Autodesk Inventor part; units mm, degrees
ref_plane "YZ Plane" through (0, 0, 0) normal (1, 0, 0) x (0, 1, 0)
ref_plane "XZ Plane" through (0, 0, 0) normal (0, 1, 0) x (-1, 0, 0)
ref_plane "XY Plane" through (0, 0, 0) normal (0, 0, 1) x (1, 0, 0)
sketch "Sketch1" plane through (0, 0, 0) normal (0, 1, 0) x (-1, 0, 0)
  line L0 (15.3914, 31.136) -> (0.1514, 31.136)
  line L1 (0.1514, 31.136) -> (0.1514, 15.896)
  line L2 (0.1514, 15.896) -> (15.3914, 15.896)
  line L3 (15.3914, 15.896) -> (15.3914, 31.136)
  point P0 (0, 0)
  dimension "d0" = 15.24
  dimension "d1" = 15.24
extrude "Extrusion1" add sketch "Sketch1" along normal blind 7.62
sketch "Sketch2" plane through (0, 0, 0) normal (0, -1, 0) x (1, 0, 0)
  circle A0 centre (-7.8533, 23.6101) radius 3.7937
  point P0 (0, 0)
extrude "Extrusion2" add sketch "Sketch2" along normal blind 1.778
sketch "Sketch3" plane through (0, 0, 0) normal (0, -1, 0) x (1, 0, 0)
  circle A0 centre (-1.4346, 30.0524) radius 0.8632
  circle A1 centre (-1.4346, 16.9205) radius 0.8792
  circle A2 centre (-14.354, 30.0524) radius 0.8098
  circle A3 centre (-14.354, 16.9205) radius 0.7609
  point P0 (0, 0)
extrude "Extrusion3" add sketch "Sketch3" along normal blind 0.508
sketch "Sketch4" plane through (0, 7.62, 0) normal (0, 1, 0) x (1, 0, 0)
  line L0 (-15.3914, -15.896) -> (-15.3914, -31.136)
  line L1 (-15.3914, -31.136) -> (-14.9868, -31.136)
  line L2 (-14.9868, -31.136) -> (-14.9868, -30.723)
  line L3 (-14.9868, -30.723) -> (-15.3914, -30.723)
  line L4 (-15.3914, -30.723) -> (-15.3914, -31.136)
  line L5 (-0.1514, -15.896) -> (-15.3914, -15.896)
  line L6 (-15.3914, -15.896) -> (-14.9868, -15.896)
  line L7 (-14.9868, -15.896) -> (-14.9868, -16.2998)
  line L8 (-14.9868, -16.2998) -> (-15.3914, -16.2998)
  line L9 (-15.3914, -16.2998) -> (-15.3914, -15.896)
  line L10 (-0.1514, -15.896) -> (-0.5623, -15.896)
  line L11 (-0.5623, -15.896) -> (-0.5623, -16.3119)
  line L12 (-0.5623, -16.3119) -> (-0.1514, -16.3119)
  line L13 (-0.1514, -16.3119) -> (-0.1514, -15.896)
  line L14 (-15.3914, -31.136) -> (-0.1514, -31.136)
  line L15 (-0.1514, -31.136) -> (-0.5623, -31.136)
  line L16 (-0.5623, -31.136) -> (-0.5623, -30.723)
  line L17 (-0.5623, -30.723) -> (-0.1514, -30.723)
  line L18 (-0.1514, -30.723) -> (-0.1514, -31.136)
  point P0 (0, 0)
extrude "Extrusion4" add sketch "Sketch4" along normal blind 6.35
properties part number "switch"
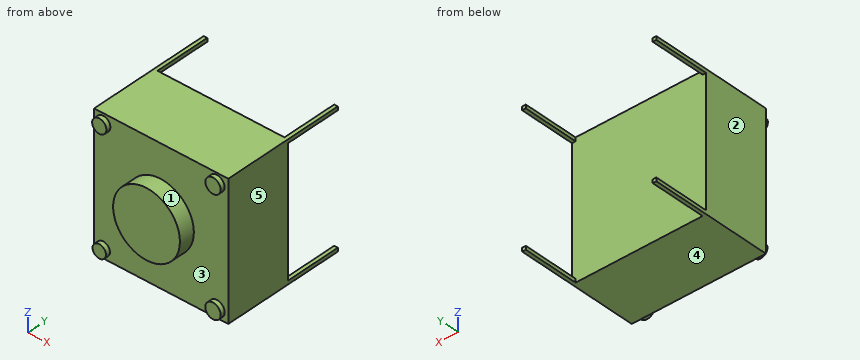
Work out the finished part from the listing and answer in its coordinate system (mm). Face numbers are marked on the shaded views. A direction names the side the tool comes from. Round coordinates to 2 decimals unless told otherwise and drop trailing zeros. Write each loop counter-clockwise with the first axis right and the second up, starting at its lowest first coordinate (ties: lowest second). Pieces come first, ordered by that corner, then holes. Notation, with made-up numbers: (87, 6.25) -> (112, 6.25) arc R29 ccw to (112, 38.25) -> close; hole circle Ø4 at (-25.5, 85.25). An arc over 180 degrees is marked (long way). Write each question's results on one line, items separated by ' | '.
Item 1: Which of the six approach directions +Z, -Z, +X, -X, +Y, -Y give full straight-line access (tool end or side, diameter ignored) to the marked faces 1 and 2?
Result set:
face 1: -Y | face 2: +Z, -Z, -X, +Y, -Y
Item 2: A cutting plane is placed at B-B, the plane x = -7.5. Determine the outline of the cut face in (y, z).
Result set:
outline: (-1.78, 19.83) -> (0, 19.83) -> (0, 15.9) -> (7.62, 15.9) -> (7.62, 31.14) -> (0, 31.14) -> (0, 27.39) -> (-1.78, 27.39) -> close
Item 3: The mould has two halves that part along Z. Classify the marked faces 3, 4 and 5: +Z half, -Z half, draft (parallel to the pull), parting line (faces both ways), or undercut.
Result set:
face 3: undercut | face 4: -Z half | face 5: draft
Item 4: A cutting plane is placed at C-C, the plane z = 29.5. Determine the outline of the cut face in (x, y), plus the area to 3 significant figures.
Result set:
outline: (-15.39, 0) -> (-14.95, 0) -> (-14.95, -0.51) -> (-13.76, -0.51) -> (-13.76, 0) -> (-2.1, 0) -> (-2.1, -0.51) -> (-0.77, -0.51) -> (-0.77, 0) -> (-0.15, 0) -> (-0.15, 7.62) -> (-15.39, 7.62) -> close | area: 117 mm^2
Item 5: A cutting plane is placed at A-A, the plane y = 11. Determine the outline of the cut face in (x, z), plus the area to 3 significant figures.
Result set:
outline: (-15.39, 15.9) -> (-14.99, 15.9) -> (-14.99, 16.3) -> (-15.39, 16.3) -> close; (-15.39, 30.72) -> (-14.99, 30.72) -> (-14.99, 31.14) -> (-15.39, 31.14) -> close; (-0.56, 15.9) -> (-0.15, 15.9) -> (-0.15, 16.31) -> (-0.56, 16.31) -> close; (-0.56, 30.72) -> (-0.15, 30.72) -> (-0.15, 31.14) -> (-0.56, 31.14) -> close | area: 0.671 mm^2
Item 6: Find the intervals of material crossed by line 1 along Y through (x, z) = (-8.5, 30); line 2 along Z through (x, y) = (-6.5, -0.5); line 3 along X through (y, z) = (-0.5, 27), in increasing order. Write a range as [from, to].
Result set:
line 1: [0, 7.62] | line 2: [20.07, 27.15] | line 3: [-9.56, -6.15]
Item 7: A cutting plane is placed at D-D, the plane x = -10.5. Determine the outline of the cut face in (y, z).
Result set:
outline: (-1.78, 20.89) -> (0, 20.89) -> (0, 15.9) -> (7.62, 15.9) -> (7.62, 31.14) -> (0, 31.14) -> (0, 26.33) -> (-1.78, 26.33) -> close
Item 8: Flat-ended cylindrical pins translate along their axes: P1, Ø1.5, axis at x = -12.5, z = 25, coming from the -Y side; P2, Ø1.9, axis at x = -1.5, z = 30.5, coming from the -Y side; P3, Ø5, axis at x = -5, z = 29, coming from the +Y side. Find the tip coordinate at first contact, or state that the pin passes through.
Result set:
P1: y = 0 | P2: y = -0.51 | P3: y = 7.62
